Verification items for the finished model (mm, model axes). A direction names the side the tool comes from. Give positions to 0.01 mm unless a question says otherwise; leave off trailing zeros. Order: outer loops, then holes, each group sorted by start corner. A loop starts at its lowest first (then second) coordinate and runs counter-clockwise, first axis right, second up. Notation, with made-up numbers: (78.5, -38) -> (83.5, -38) arc R34 ccw to (83.5, -5) -> close; hole circle Ø7 at (85.5, -25.75). An arc over 180 degrees is marked (long way). One line per question, with ' | ' between items. Start each with the question number.
Q1. Go/stop test with flat-tipped pins: pin 1 (12 mm diameter, centred on y = 22, z = -16, fed in from -X); pin 2 (3 mm diameter, centred on y = 10, z = 7.5, fed in from +X); pin 3 (2 mm diameter, centred on x = -12.5, y = 21.5, fed in from +Z). Record where each tip stops, or that it passes through.
Q2. Section check A-A on z = 0. Record the cut outline in (x, y), plus the area to 3 significant figures.
Q3. Material ranges on probe 1 along Y at (x, z) = (-6, -12); probe 2 along Z at (x, y) = (-10.5, 22); probe 3 along X at (y, z) = (27.5, 3), recorded low to high. Write a range as [from, to].
Q4. Section check B-B on y = 24.25. Record the cut outline in (x, z), plus the area to 3 significant figures.
Q5. Access from +Z, -Z, +X, -X, +Y, -Y to the whole of each face (thin tool, end or side, straight path). Record for faces 4 (the flat face through (0, 5, 0)), 5 (the flat face through (35.467, 15.21, 6.254)), 6 (the flat face through (-35.467, 15.21, -6.254)).
Q6. Mould release check, pull along Z, two halves, no side actions. Record for faces 1 (the flat face through (6.254, 15.21, -35.467)), 2 (the flat face through (-1, 0, -1)), 3 (the cylindrical face through (-37, 15, 0)): released by +Z, released by -Z, zero draft, split by the parting line, or undercut.
Q7. Section check C-C on x = 0. Record the cut outline in (y, z), plus the area to 3 significant figures.
from build123d import *

# Parameters (mm, degrees)
SKETCH1_R           = 37
BOSS_EXTRUDE1_DEPTH = 30
CUT_EXTRUDE1_DEPTH  = 30
SKETCH3_R           = 33
CUT_EXTRUDE2_DEPTH  = 25


with BuildPart() as part:
    # Sketch1 → Boss-Extrude1 (new body)
    with BuildSketch(Plane(origin=(0, 0, 0), x_dir=(1, 0, 0), z_dir=(0, 1, 0))):
        Circle(SKETCH1_R)
    extrude(amount=BOSS_EXTRUDE1_DEPTH)

    # Sketch2 → Cut-Extrude1 (cut)
    with BuildSketch(Plane(origin=(0, 30, 0), x_dir=(1, 0, 0), z_dir=(0, 1, 0))):
        with BuildLine():
            Line((6.424982574, 36.437886861), (6.077686218, 34.468271355))
            ThreePointArc((6.077686218, 34.468271355), (24.748737342, 24.748737342), (34.468271355, 6.077686218))
            Line((34.468271355, 6.077686218), (36.437886861, 6.424982574))
            ThreePointArc((36.437886861, 6.424982574), (26.162950904, 26.162950904), (6.424982574, 36.437886861))
        make_face()
        with BuildLine():
            Line((36.437886861, -6.424982574), (34.468271355, -6.077686218))
            ThreePointArc((34.468271355, -6.077686218), (24.748737342, -24.748737342), (6.077686218, -34.468271355))
            Line((6.077686218, -34.468271355), (6.424982574, -36.437886861))
            ThreePointArc((6.424982574, -36.437886861), (26.162950904, -26.162950904), (36.437886861, -6.424982574))
        make_face()
        with BuildLine():
            Line((-6.424982574, -36.437886861), (-6.077686218, -34.468271355))
            ThreePointArc((-6.077686218, -34.468271355), (-24.748737342, -24.748737342), (-34.468271355, -6.077686218))
            Line((-34.468271355, -6.077686218), (-36.437886861, -6.424982574))
            ThreePointArc((-36.437886861, -6.424982574), (-26.162950904, -26.162950904), (-6.424982574, -36.437886861))
        make_face()
        with BuildLine():
            Line((-36.437886861, 6.424982574), (-34.468271355, 6.077686218))
            ThreePointArc((-34.468271355, 6.077686218), (-24.748737342, 24.748737342), (-6.077686218, 34.468271355))
            Line((-6.077686218, 34.468271355), (-6.424982574, 36.437886861))
            ThreePointArc((-6.424982574, 36.437886861), (-26.162950904, 26.162950904), (-36.437886861, 6.424982574))
        make_face()
    extrude(amount=-CUT_EXTRUDE1_DEPTH, mode=Mode.SUBTRACT)

    # Sketch3 → Cut-Extrude2 (cut)
    with BuildSketch(Plane(origin=(0, 30, 0), x_dir=(1, 0, 0), z_dir=(0, 1, 0))):
        Circle(SKETCH3_R)
    extrude(amount=-CUT_EXTRUDE2_DEPTH, mode=Mode.SUBTRACT)


solid = part.part
Filled in:
1) pin 1: x = -33.54 | pin 2: x = 36.51 | pin 3: z = 33.06
2) outline: (-37, 0) -> (37, 0) -> (37, 30) -> (33, 30) -> (33, 5) -> (-33, 5) -> (-33, 30) -> (-37, 30) -> close | area: 570 mm²
3) probe 1: [0, 5] | probe 2: [-33.39, -31.28], [31.28, 33.39] | probe 3: [-36.88, -32.86], [32.86, 36.88]
4) outline: (-36.44, -6.42) -> (-34.47, -6.08) arc R35 ccw to (-6.08, -34.47) -> (-6.42, -36.44) arc R37 ccw to (6.42, -36.44) -> (6.08, -34.47) arc R35 ccw to (34.47, -6.08) -> (36.44, -6.42) arc R37 ccw to (36.44, 6.42) -> (34.47, 6.08) arc R35 ccw to (6.08, 34.47) -> (6.42, 36.44) arc R37 ccw to (-6.42, 36.44) -> (-6.08, 34.47) arc R35 ccw to (-34.47, 6.08) -> (-36.44, 6.42) arc R37 ccw to start; hole circle Ø66 at (0, 0) | area: 528 mm²
5) face 4: +Y | face 5: +Z, +Y, -Y | face 6: -Z, +Y, -Y
6) face 1: undercut | face 2: zero draft | face 3: split by the parting line
7) outline: (0, -37) -> (30, -37) -> (30, -33) -> (5, -33) -> (5, 33) -> (30, 33) -> (30, 37) -> (0, 37) -> close | area: 570 mm²
